from build123d import *

# Parameters (mm, degrees)
F0_R     = 10
F1_DEPTH = 2
F2_R     = 5.5
F3_DEPTH = 1
F4_R     = 4.15
F5_DEPTH = 3.5
F6_R     = 2.5
F7_DEPTH = 10
F8_R     = 1


with BuildPart() as f1:
    # F0 (on Top) → F1 (new body)
    with BuildSketch(Plane.XY):
        Circle(F0_R)
    extrude(amount=F1_DEPTH)

    # F2 (on face) → F3 (join)
    with BuildSketch(Plane.XY.offset(2)):
        Circle(F2_R)
    extrude(amount=F3_DEPTH)

    # F4 (on face) → F5 (join)
    with BuildSketch(Plane.XY.offset(3)):
        Circle(F4_R)
    extrude(amount=F5_DEPTH)

    # F6 (on face) → F7 (cut)
    with BuildSketch(Plane.XY.offset(6.5)):
        Circle(F6_R)
    extrude(amount=-F7_DEPTH, mode=Mode.SUBTRACT)

    # F8
    f8_edges = [f1.edges().sort_by_distance(p)[0] for p in [
        (-10, 0, 0),
    ]]
    fillet(f8_edges, radius=F8_R)


solid = f1.part
Model file for the job. Use its own axes, mm. A direction names the side the tool comes from. Give positions to 0.01 mm unless a question says otherwise; leave off trailing zeros. Order: outer loops, then holes, each group sorted by start corner. A loop starts at its lowest first (then second) coordinate and runs counter-clockwise, first axis right, second up. Notation, with made-up numbers: M -12.75,-31.5 L 19.25,-31.5 A25 cw 19.25,3.5 Z; hole C 34,6.25 d5. An arc over 180 degrees is marked long. Put each result on its own line as item: value. Start each with the question number.
(1) Band-saw the part on A-A on x = 0. Give the cut face in (y, z).
(2) Band-saw the part on D-D on z = 4.75. Give the cut face in (x, y), then the cut area to 3 significant figures.
(3) Pin check, flat tips, straight feed: pin 1 Ø2 at (x, y) = (-8, 2.5) entering from +Z; pin 2 Ø5 at (x, y) = (6, -5) entering from +Z; pin 3 Ø3 at (x, y) = (0, 0) entering from +Z; pin 4 Ø1.5 at (x, z) = (-1.5, 5.5) entering from -Y. Stop position of each tip, or through.
(4) Pull direction Y, two halves, no side cores. Call faces 3 (the face through (-0.9, -4.05, 4.73)), 4 (the face through (-0.54, -2.44, 3.3)), 5 (the face through (2, -2, 6.5)): released by +Y, released by -Y, zero draft, split by the parting line, or undercut.
(5) Tool access for faces 1 (the face through (2, -2, 0)), 2 (the face through (-2, 4, 3)): list every direction of +Z, -Z, +X, -X, +Y, -Y with a clear straight run to the whole face (end or side of a thin tool).
(6) Band-saw the part on C-C on z = 1.5. Give the cut face in (x, y).
(7) Drill centre lines: L1, parallel to Y at x = 0, z = 5.25; L2, parallel to Y at x = 0, z = 1.75; L3, parallel to Z at x = -5.5, y = 2.5. Where is each one in solid material? Low to high. Write a range as [from, to].
Results below:
1. outline: M -10,1 A1 ccw -9,0 L -2.5,0 L -2.5,6.5 L -4.15,6.5 L -4.15,3 L -5.5,3 L -5.5,2 L -10,2 Z; M 2.5,0 L 9,0 A1 ccw 10,1 L 10,2 L 5.5,2 L 5.5,3 L 4.15,3 L 4.15,6.5 L 2.5,6.5 Z
2. outline: C 0,0 d8.3; hole C 0,0 d5
2. area: 34.5 mm2
3. pin 1: stops at z = 2
3. pin 2: stops at z = 3
3. pin 3: passes through
3. pin 4: stops at y = -4.08
4. face 3: split by the parting line
4. face 4: undercut
4. face 5: zero draft
5. face 1: -Z, +X, -X, +Y, -Y
5. face 2: +Z
6. outline: C 0,0 d20; hole C 0,0 d5
7. L1: y = [-4.15, -2.5], [2.5, 4.15]
7. L2: y = [-10, -2.5], [2.5, 10]
7. L3: z = [0, 2]
